For this review, take the finished solid that the model builds, in its own axes (mm). Round coordinates to 2 decimals unless told otherwise and drop trailing zeros. Order: outer loops, then holes, each group sorted by start corner. A loop starts at its lowest first (then second) coordinate and runs counter-clockwise, first axis right, second up. Notation, with made-up numbers: (21.25, 25.25) -> (43.25, 25.25) arc R27 cw to (43.25, 41.25) -> close; hole circle Ø3 at (-17.5, 11). An arc over 180 degrees is marked (long way). Answer in a Markdown table with one row per item.
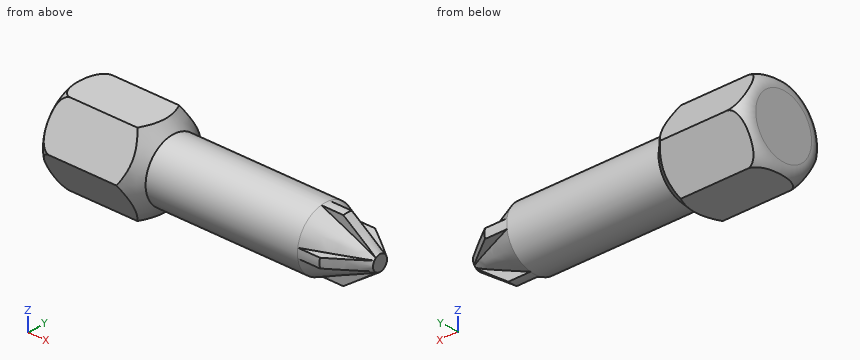
```python
from build123d import *
from build123d.topology import SkipClean

# Parameters (mm, degrees)
SKETCH2_OUTSIDE_W   = 53.726
SKETCH2_OUTSIDE_H   = 53.726
CUT_EXTRUDE2_DEPTH  = 100
BOSS_EXTRUDE1_DEPTH = 18


with BuildPart() as part:
    # Sketch1 → Revolve1 (revolve)
    with BuildSketch(Plane(origin=(0, 0, 0), x_dir=(1, 0, 0), z_dir=(0, 0, -1)), mode=Mode.PRIVATE) as revolve1_sk:
        with BuildLine():
            Line((0, 0), (0, 10))
            ThreePointArc((0, 10), (1.464466094, 13.535533906), (5, 15))
            Line((5, 15), (27, 15))
            Line((27, 15), (32, 10))
            Line((32, 10), (82, 10))
            Line((82, 10), (100, 2.5))
            Line((100, 2.5), (100, 0))
            Line((100, 0), (0, 0))
        make_face()
    revolve(revolve1_sk.sketch.rotate(Axis((-28.136645963, 0, 0), (1, 0, 0)), 270), axis=Axis((-28.136645963, 0, 0), (1, 0, 0)))  # turned: the seam where the file's is

    # Sketch2 outside → Cut-Extrude2 (cut)
    with BuildSketch(Plane.ZY):
        Rectangle(SKETCH2_OUTSIDE_W, SKETCH2_OUTSIDE_H)
        Polygon((12.990381057, -7.5), (12.990381057, 7.5), (0, 15), (-12.990381057, 7.5), (-12.990381057, -7.5), (0, -15), align=None, mode=Mode.SUBTRACT)
    extrude(amount=-CUT_EXTRUDE2_DEPTH, mode=Mode.SUBTRACT)

    # Sketch5 → Boss-Extrude1 (add)
    with SkipClean():  # keep this step's faces unmerged: merging them makes the solid invalid here
        with BuildSketch(Plane(origin=(100, 0, 0), x_dir=(0, 0, -1), z_dir=(1, 0, 0))):
            with BuildLine():
                Line((-1.5, 2), (-1.5, 9.886859967))
                ThreePointArc((-1.5, 9.886859967), (0, 10), (1.5, 9.886859967))
                Line((1.5, 9.886859967), (1.5, 2))
                ThreePointArc((1.5, 2), (1.767766953, 1.767766953), (2, 1.5))
                Line((2, 1.5), (9.886859967, 1.5))
                ThreePointArc((9.886859967, 1.5), (10, 0), (9.886859967, -1.5))
                Line((9.886859967, -1.5), (2, -1.5))
                ThreePointArc((2, -1.5), (1.767766953, -1.767766953), (1.5, -2))
                Line((1.5, -2), (1.5, -9.886859967))
                ThreePointArc((1.5, -9.886859967), (0, -10), (-1.5, -9.886859967))
                Line((-1.5, -9.886859967), (-1.5, -2))
                ThreePointArc((-1.5, -2), (-1.767766953, -1.767766953), (-2, -1.5))
                Line((-2, -1.5), (-9.886859967, -1.5))
                ThreePointArc((-9.886859967, -1.5), (-10, 0), (-9.886859967, 1.5))
                Line((-9.886859967, 1.5), (-2, 1.5))
                ThreePointArc((-2, 1.5), (-1.767766953, 1.767766953), (-1.5, 2))
            make_face()
        extrude(amount=-BOSS_EXTRUDE1_DEPTH)

    # Sketch6 → Cut-Revolve1 (revolve, cut)
    with SkipClean():  # keep this step's faces unmerged: merging them makes the solid invalid here
        with BuildSketch(Plane.XY, mode=Mode.PRIVATE) as cut_revolve1_sk:
            Polygon((100, 2.5), (100, 10), (89.288889949, 10), align=None)
        revolve(cut_revolve1_sk.sketch.rotate(Axis((100, 0, 0), (1, 0, 0)), 90), axis=Axis((100, 0, 0), (1, 0, 0)), mode=Mode.SUBTRACT)  # turned: the seam where the file's is


solid = part.part
```
Q1. Take a section at B-B, the plane x = 91. Write out the cut boundary in (y, z), then the cut area to 3 significant figures.
Answer key:
| item | result |
|---|---|
| outline | (-8.67, -1.5) -> (-6.07, -1.5) arc R6.25 ccw to (-1.5, -6.07) -> (-1.5, -8.67) arc R8.8 ccw to (1.5, -8.67) -> (1.5, -6.07) arc R6.25 ccw to (6.07, -1.5) -> (8.67, -1.5) arc R8.8 ccw to (8.67, 1.5) -> (6.07, 1.5) arc R6.25 ccw to (1.5, 6.07) -> (1.5, 8.67) arc R8.8 ccw to (-1.5, 8.67) -> (-1.5, 6.07) arc R6.25 ccw to (-6.07, 1.5) -> (-8.67, 1.5) arc R8.8 ccw to start |
| area | 154 mm^2 |
Q2. To check wall thickness, follow probe 1 along Z at (x, y) = (89, -8); probe 2 along Y at (x, z) = (85, 0); probe 3 along Y at (x, z) = (78, 6.75). State the ranges of each line that lie inside material, in increasing order.
Answer key:
| item | result |
|---|---|
| probe 1 | z = -1.5 to 1.5 |
| probe 2 | y = -10 to 10 |
| probe 3 | y = -7.38 to 7.38 |
Q3. Take a section at C-C, the plane x = 53. Write out the cut boundary in (y, z), then the cut area to 3 significant figures.
Answer key:
| item | result |
|---|---|
| outline | circle Ø20 at (0, 0) |
| area | 314 mm^2 |
Q4. Take a section at A-A, the plane y = 0. Write out the cut boundary in (x, z).
Answer key:
| item | result |
|---|---|
| outline | (0, -10) arc R5 ccw to (0.99, -12.99) -> (29.01, -12.99) -> (32, -10) -> (89.29, -10) -> (100, -2.5) -> (100, 2.5) -> (89.29, 10) -> (32, 10) -> (29.01, 12.99) -> (0.99, 12.99) arc R5 ccw to (0, 10) -> close |
Q5. Clearance check with flat-ended pins moving along their axes: pin 1 Ø4 at (x, y) = (92, -8) entering from +Z; pin 2 Ø8.5 at (x, z) = (88.5, -7.5) entering from +Y; pin 3 Ø8 at (y, z) = (-4.5, -6.5) entering from -X; pin 4 Ø2 at (x, z) = (71.5, -6) entering from +Y. State where each tip first meets the part, or that it passes through.
Answer key:
| item | result |
|---|---|
| pin 1 | stops at z = 1.5 |
| pin 2 | stops at y = 7.28 |
| pin 3 | stops at x = 0 |
| pin 4 | stops at y = 8.66 |
Q6. Take a section at D-D, the plane x = 23.5. Write out the cut boundary in (y, z).
Answer key:
| item | result |
|---|---|
| outline | (-15, 0) -> (-7.5, -12.99) -> (7.5, -12.99) -> (15, 0) -> (7.5, 12.99) -> (-7.5, 12.99) -> close |
